Work out the finished part from the listing and answer in its coordinate system (mm). A direction names the side the tool comes from. Round coordinates to 2 decimals unless told otherwise and drop trailing zeros. Order: outer loops, then holes, each group sorted by start corner. A loop starts at its lowest first (then second) coordinate and runs counter-clockwise, first axis right, second up. Notation, with made-up numbers: (-23, 56.5) - (-13, 56.5) arc R34 ccw to (-13, 89.5) - close; hole circle Ø9 at (86, 26.25). An arc over 180 degrees is marked (long way). Put each result on its own line as item: value.
```python
from build123d import *

# Parameters (mm, degrees)
SKIZZE1_R                       = 1.5
AUFSATZ_LINEAR_AUSTRAGEN1_DEPTH = 2
SKIZZE2_OUTSIDE_W               = 12.684
SKIZZE2_OUTSIDE_H               = 14.684
SCHNITT_LINEAR_AUSTRAGEN1_DEPTH = 1.1


with BuildPart() as part:
    # Skizze1 → Aufsatz-Linear austragen1 (new body, symmetric)
    with BuildSketch(Plane.XY):
        with BuildLine():
            Line((-4, 0), (-4, 6))
            Line((-4, 6), (4, 6))
            Line((4, 6), (4, 0))
            ThreePointArc((4, 0), (0, -4), (-4, 0))
        make_face()
        Circle(SKIZZE1_R, mode=Mode.SUBTRACT)
    extrude(amount=AUFSATZ_LINEAR_AUSTRAGEN1_DEPTH, both=True)

    # Skizze2 outside → Schnitt-Linear austragen1 (cut, symmetric)
    with BuildSketch(Plane.XY):
        with Locations((0, 1)):
            Rectangle(SKIZZE2_OUTSIDE_W, SKIZZE2_OUTSIDE_H)
        with BuildLine():
            Line((-3, 6), (3, 6))
            Line((3, 6), (3, 0))
            ThreePointArc((3, 0), (0, -3), (-3, 0))
            Line((-3, 0), (-3, 6))
        make_face(mode=Mode.SUBTRACT)
    extrude(amount=SCHNITT_LINEAR_AUSTRAGEN1_DEPTH, both=True, mode=Mode.SUBTRACT)


solid = part.part
```
1) A cutting plane is placed at C-C on y = 2.5. Write down the section's boundary in (x, z), then the cut area to 3 significant figures.
Findings below:
outline: (-4, -2) - (4, -2) - (4, -1.1) - (3, -1.1) - (3, 1.1) - (4, 1.1) - (4, 2) - (-4, 2) - (-4, 1.1) - (-3, 1.1) - (-3, -1.1) - (-4, -1.1) - close
area: 27.6 mm2
2) A cutting plane is placed at D-D on z = -1.65. Write down the section's boundary in (x, y), then the cut area to 3 significant figures.
Findings below:
outline: (-4, 0) arc R4 ccw to (4, 0) - (4, 6) - (-4, 6) - close; hole circle Ø3 at (0, 0)
area: 66.1 mm2
3) Given pin 1 Ø1.1 at (y, z) = (4, 0) entering from +X, flat-ended and moving along its own axis, determine where the tip first touches the part or whether it passes through.
Findings below:
pin 1: stops at x = 3
4) For a pull along X with two mould halves and no side action, classify faces 6 (the flat face through (-4, 3, 1.6)), 7 (the cylindrical face through (0.1, -4, -1.5)), 8 (the cylindrical face through (-1.5, 0.07, -0.03)) as pulls with the +X half, pulls with the -X half, needs draft (parallel to the pull), parting line crosses it, or undercut.
Findings below:
face 6: pulls with the -X half
face 7: parting line crosses it
face 8: undercut
5) Straight lines are drawn through the part: L1, parallel to Y at x = 0, z = -0.25; L2, parallel to X at y = 3.5, z = 0; L3, parallel to Y at x = -1, z = -1.05. For each, find the intervals that lie inside material, in ascending order. Write a range as from..to.
Findings below:
L1: y = -3..-1.5, 1.5..6
L2: x = -3..3
L3: y = -2.83..-1.12, 1.12..6
6) For faces 1 (the flat face through (3, -1, -1.1)), 2 (the flat face through (-3, 3, 0)), 3 (the flat face through (3, 3, 0)), 4 (the flat face through (0, 6, 0)), 5 (the cylindrical face through (0.1, -4, 1.6)), determine the directions among +Z, -Z, +X, -X, +Y, -Y from which every point of the face is accessible in a straight line to the end or side of a thin tool.
Findings below:
face 1: -Y
face 2: -X, +Y, -Y
face 3: +X, +Y, -Y
face 4: +Z, -Z, +X, -X, +Y
face 5: +Z, -Z, -Y
7) A cutting plane is placed at A-A on x = 0. Write down the section's boundary in (y, z), then the cut area to 3 significant figures.
Findings below:
outline: (-4, -2) - (-1.5, -2) - (-1.5, 2) - (-4, 2) - (-4, 1.1) - (-3, 1.1) - (-3, -1.1) - (-4, -1.1) - close; (1.5, -2) - (6, -2) - (6, 2) - (1.5, 2) - close
area: 25.8 mm2
8) A cutting plane is placed at B-B on z = -0.25. Write down the section's boundary in (x, y).
Findings below:
outline: (-3, 0) arc R3 ccw to (3, 0) - (3, 6) - (-3, 6) - close; hole circle Ø3 at (0, 0)
